For this review, take the finished solid that the model builds, in its own axes (mm). Face numbers are marked on the shaded views. A direction names the side the tool comes from. Round coordinates to 2 decimals unless told otherwise and drop trailing zeros. Write each loop counter-clockwise with the first axis right and the second up, starting at its lowest first coordinate (ties: lowest second). Pieces come first, ordered by that corner, then holes. Notation, with made-up numbers: (46.25, -4.75) -> (59.25, -4.75) arc R19 cw to (59.25, 20.25) -> close; hole circle Ø10 at (88.25, -10.75). An arc over 180 degrees is marked (long way). Answer in a Markdown table with one row per item.
from build123d import *

# Parameters (mm, degrees)
F1_DEPTH = 5.08
F2_DEPTH = 5.0292
F3_W     = 11.43
F3_H     = 3.81
F4_DEPTH = 1.016


with BuildPart() as f1:
    # F0 (on Top) → F1 (new body)
    with BuildSketch(Plane.XY):
        with BuildLine():
            ThreePointArc((1.524, 0), (1.4720709593, -0.3944402247), (1.3198227154, -0.762))
            Line((1.3198227154, -0.762), (1.8837144157, -0.762))
            ThreePointArc((1.8837144157, -0.762), (1.9945841287, -0.3881470773), (2.032, 0))
            Line((2.032, 0), (1.524, 0))
        make_face()
        with BuildLine():
            Line((1.8837144157, 0.762), (1.3198227154, 0.762))
            ThreePointArc((1.3198227154, 0.762), (1.4720709593, 0.3944402247), (1.524, 0))
            Line((1.524, 0), (2.032, 0))
            ThreePointArc((2.032, 0), (1.9945841287, 0.3881470773), (1.8837144157, 0.762))
        make_face()
        Polygon((19.812, 0.2309090909), (13.97, 0.762), (13.97, 0), (19.812, 0), align=None)
        Polygon((13.97, 0), (13.97, -0.762), (19.812, -0.2309090909), (19.812, 0), align=None)
        Polygon((22.352, 0), (19.812, 0.2309090909), (19.812, 0), align=None)
        Polygon((19.812, 0), (19.812, -0.2309090909), (22.352, 0), align=None)
        with BuildLine():
            ThreePointArc((0, -1.524), (-1.524, 0), (0, 1.524))
            Line((0, 1.524), (0, 2.032))
            ThreePointArc((0, 2.032), (-2.032, 0), (0, -2.032))
            Line((0, -2.032), (0, -1.524))
        make_face()
        with BuildLine():
            ThreePointArc((0.4517456439, -1.4555074281), (0.2284542401, -1.5067795659), (0, -1.524))
            Line((0, -1.524), (0, -2.032))
            Line((0, -2.032), (0.3664262295, -1.9986885246))
            ThreePointArc((0.3664262295, -1.9986885246), (0.4091799306, -1.9903757897), (0.4517456439, -1.9811486247))
            Line((0.4517456439, -1.9811486247), (0.4517456439, -1.4555074281))
        make_face()
        with BuildLine():
            Line((0, 2.032), (0, 1.524))
            ThreePointArc((0, 1.524), (0.2284542401, 1.5067795659), (0.4517456439, 1.4555074281))
            Line((0.4517456439, 1.4555074281), (0.4517456439, 1.9811486247))
            ThreePointArc((0.4517456439, 1.9811486247), (0.4091799306, 1.9903757897), (0.3664262295, 1.9986885246))
            Line((0.3664262295, 1.9986885246), (0, 2.032))
        make_face()
        with BuildLine():
            Line((0.4517456439, 1.9811486247), (0.4517456439, 1.4555074281))
            ThreePointArc((0.4517456439, 1.4555074281), (0.9512369584, 1.1906822619), (1.3198227154, 0.762))
            Line((1.3198227154, 0.762), (1.8837144157, 0.762))
            ThreePointArc((1.8837144157, 0.762), (1.3172601356, 1.5472070757), (0.4517456439, 1.9811486247))
        make_face()
        with BuildLine():
            ThreePointArc((1.3198227154, -0.762), (0.9512369584, -1.1906822619), (0.4517456439, -1.4555074281))
            Line((0.4517456439, -1.4555074281), (0.4517456439, -1.9811486247))
            ThreePointArc((0.4517456439, -1.9811486247), (1.3172601356, -1.5472070757), (1.8837144157, -0.762))
            Line((1.8837144157, -0.762), (1.3198227154, -0.762))
        make_face()
        with BuildLine():
            Line((13.97, 0.762), (1.8837144157, 0.762))
            ThreePointArc((1.8837144157, 0.762), (1.9945841287, 0.3881470773), (2.032, 0))
            Line((2.032, 0), (13.97, 0))
            Line((13.97, 0), (13.97, 0.762))
        make_face()
        with BuildLine():
            ThreePointArc((2.032, 0), (1.9945841287, -0.3881470773), (1.8837144157, -0.762))
            Line((1.8837144157, -0.762), (13.97, -0.762))
            Line((13.97, -0.762), (13.97, 0))
            Line((13.97, 0), (2.032, 0))
        make_face()
        Polygon((22.352, 0.2309090909), (19.812, 0.2309090909), (22.352, 0), align=None)
        Polygon((22.352, 0), (19.812, -0.2309090909), (22.352, -0.2309090909), align=None)
    extrude(amount=F1_DEPTH)

    # F0 (on Top) → F2 (join)
    with BuildSketch(Plane.XY):
        with BuildLine():
            ThreePointArc((1.524, 0), (1.4720709593, -0.3944402247), (1.3198227154, -0.762))
            Line((1.3198227154, -0.762), (1.8837144157, -0.762))
            ThreePointArc((1.8837144157, -0.762), (1.9945841287, -0.3881470773), (2.032, 0))
            Line((2.032, 0), (1.524, 0))
        make_face()
        with BuildLine():
            Line((0, 2.032), (0, 1.524))
            ThreePointArc((0, 1.524), (0.2284542401, 1.5067795659), (0.4517456439, 1.4555074281))
            Line((0.4517456439, 1.4555074281), (0.4517456439, 1.9811486247))
            ThreePointArc((0.4517456439, 1.9811486247), (0.4091799306, 1.9903757897), (0.3664262295, 1.9986885246))
            Line((0.3664262295, 1.9986885246), (0, 2.032))
        make_face()
        with BuildLine():
            ThreePointArc((0, -1.524), (-1.524, 0), (0, 1.524))
            Line((0, 1.524), (0, 2.032))
            ThreePointArc((0, 2.032), (-2.032, 0), (0, -2.032))
            Line((0, -2.032), (0, -1.524))
        make_face()
    extrude(amount=F2_DEPTH)

    # F3 (on Top) → F4 (join)
    with BuildSketch(Plane.XY):
        with Locations((7.7741611749, 0)):
            Rectangle(F3_W, F3_H)
    extrude(amount=F4_DEPTH)


solid = f1.part
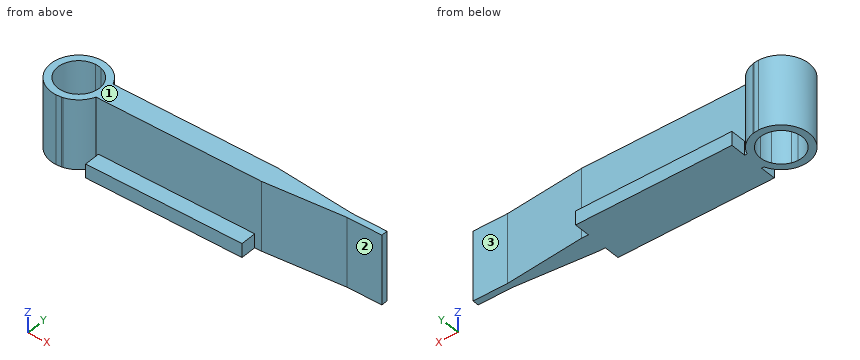
1) Consider section C-C on y = 1.25. State the section outline as (x, z) points.
Solved:
| item | result |
|---|---|
| outline | (-1.6, 0) -> (-0.87, 0) -> (-0.87, 5.08) -> (-1.6, 5.08) -> close; (0.87, 0) -> (1.6, 0) -> (1.6, 5.08) -> (0.87, 5.08) -> close; (2.06, 0) -> (13.49, 0) -> (13.49, 1.02) -> (2.06, 1.02) -> close |
2) For the marked faces 1, 2 and 3, list the 3-axis set-ups (+Z, -Z, +X, -X, +Y, -Y) from which the entire face can be reached by the end or side of a thin tool; tool diameter is ignored.
Solved:
| item | result |
|---|---|
| face 1 | +Z, +X, -X, +Y, -Y |
| face 2 | +Z, -Z, +X, -Y |
| face 3 | +Z, -Z, +X, +Y |
3) Consider section D-D on y = -1. State the section outline as (x, z) points, then the cut area to 3 significant figures.
Solved:
| item | result |
|---|---|
| outline | (-1.77, 0) -> (-1.15, 0) -> (-1.15, 5.08) -> (-1.77, 5.08) -> close; (1.15, 0) -> (1.77, 0) -> (1.77, 5.08) -> (1.15, 5.08) -> close; (2.06, 0) -> (13.49, 0) -> (13.49, 1.02) -> (2.06, 1.02) -> close |
| area | 17.9 mm² |
4) Clearance check with flat-ended pins moving along their axes: pin 1 Ø0.8 at (x, z) = (20.5, 3.5) entering from +Y; pin 2 Ø0.5 at (x, z) = (7.5, 0.5) entering from +Y (3 decimals); pin 3 Ø0.5 at (y, z) = (1.5, 0.5) entering from -X. State where each tip first meets the part, or that it passes through.
Solved:
| item | result |
|---|---|
| pin 1 | y = 0.23 |
| pin 2 | y = 1.905 |
| pin 3 | x = -1.6 |
5) Consider section A-A on z = 4.05. State the section outline as (x, y) points, then the cut area to 3 significant figures.
Solved:
| item | result |
|---|---|
| outline | (0, -2.03) -> (0.37, -2) arc R2.03 ccw to (1.88, -0.76) -> (13.97, -0.76) -> (19.81, -0.23) -> (22.35, -0.23) -> (22.35, 0.23) -> (19.81, 0.23) -> (13.97, 0.76) -> (1.88, 0.76) arc R2.03 ccw to (0.37, 2) -> (0, 2.03) arc R2.03 ccw to start; hole circle Ø3.05 at (0, 0) |
| area | 30.9 mm² |
6) For line 1 (X direction, y = -0.05, z = 1.7); line 2 (X direction, y = -1.2, z = 0.3); line 3 (X direction, y = -0.95, z = 0.45), list the stretches that pass through material, from the lowest coordinate up. Write a range as [from, to].
Solved:
| item | result |
|---|---|
| line 1 | [-2.03, -1.52], [1.52, 22.35] |
| line 2 | [-1.64, -0.94], [0.94, 1.64], [2.06, 13.49] |
| line 3 | [-1.8, -1.19], [1.19, 1.8], [2.06, 13.49] |
7) Consider section B-B on x = 9. State the section outline as (y, z) points (3 decimals).
Solved:
| item | result |
|---|---|
| outline | (-1.905, 0) -> (1.905, 0) -> (1.905, 1.016) -> (0.762, 1.016) -> (0.762, 5.08) -> (-0.762, 5.08) -> (-0.762, 1.016) -> (-1.905, 1.016) -> close |
